from build123d import *

# Parameters (mm, degrees)
F0_R          = 14.5
F2_R          = 12.5
F5_R          = 10.8
F4_R          = 12.8
F8_R          = 14.5
F8_R_2        = 12.25
F9_DEPTH      = 0.5
F10_DEPTH     = 0.5
F11_R         = 0.2
F13_R         = 14
F13_R_2       = 12.2
F14_DEPTH     = 0.5
F15_DEPTH     = 0.5
F16_W         = 3
F16_H         = 15
F16_H_2       = 3
F16_W_2       = 15
F17_DEPTH     = 10
F18_T2_ANGLE  = 82.921707092
F18_T4_ANGLE  = 82.921707092
F18_T6_ANGLE  = 82.921707092
F18_T8_ANGLE  = 82.921707092
F18_T10_ANGLE = 82.921707092
F18_T12_ANGLE = 82.921707092
F18_T14_ANGLE = 82.921707092
F18_T16_ANGLE = 82.921707092


# Not quite as in the source:
# - a fillet or chamfer that OpenCascade refuses, or shapes differently, is made with other operations: its cross-section is extruded or revolved along the edge and cut away or added
# - a feature of the source that left no trace in its solid (it failed there, or was rolled back) is left out


with BuildPart() as f3:
    # F0 (on Top) → F3 section 0
    with BuildSketch(Plane.XY):
        Circle(F0_R)
    # F2 (on offset) → F3 section 1
    with BuildSketch(Plane.XY.offset(90)):
        Circle(F2_R)
    loft()

    # F5 (on face) → F6 section 0
    with BuildSketch(Plane.XY.offset(90)):
        Circle(F5_R)
    # F4 (on Top) → F6 section 1
    with BuildSketch(Plane.XY):
        Circle(F4_R)
    loft(mode=Mode.SUBTRACT)

    # F8 (on offset) → F9 (cut)
    with BuildSketch(Plane.XY.offset(81)):
        Circle(F8_R)
        Circle(F8_R_2, mode=Mode.SUBTRACT)
    extrude(amount=F9_DEPTH, mode=Mode.SUBTRACT)

    # F8 (on offset) → F10 (cut)
    with BuildSketch(Plane.XY.offset(81)):
        Circle(F8_R)
        Circle(F8_R_2, mode=Mode.SUBTRACT)
    extrude(amount=-F10_DEPTH, mode=Mode.SUBTRACT)

    # F11
    f11_edges = [f3.edges().sort_by_distance(p)[0] for p in [
        (-12.711111, 0, 80.5),
        (-12.688889, 0, 81.5),
    ]]
    fillet(f11_edges, radius=F11_R)

    # F13 (on offset) → F14 (join)
    with BuildSketch(Plane.XY.offset(3)):
        Circle(F13_R)
        Circle(F13_R_2, mode=Mode.SUBTRACT)
    extrude(amount=F14_DEPTH)

    # F13 (on offset) → F15 (join)
    with BuildSketch(Plane.XY.offset(3)):
        Circle(F13_R)
        Circle(F13_R_2, mode=Mode.SUBTRACT)
    extrude(amount=F15_DEPTH)

    # F16 (on face) → F17 (cut)
    with BuildSketch(Plane.XY):
        with Locations((0, 9)):
            Rectangle(F16_W, F16_H)
        Rectangle(F16_W, F16_H_2)
        with Locations((-9, 0)):
            Rectangle(F16_W_2, F16_H_2)
        with Locations((9, 0)):
            Rectangle(F16_W_2, F16_H_2)
        with Locations((0, -9)):
            Rectangle(F16_W, F16_H)
    extrude(amount=F17_DEPTH, mode=Mode.SUBTRACT)

    # F18: fillet of radius 0.3 on 8 edges, made by hand

    # F18_s1 → F18_t2 (revolve, cut)
    with BuildSketch(Plane(origin=(0, 0, 0), x_dir=(0, 0, 1), z_dir=(-0.0617304854, 0.998092855, 0))):
        with BuildLine():
            ThreePointArc((3.3, -12.2), (3.0878679656, -12.2878679656), (3, -12.5))
            Line((3, -12.5), (3, -12.2))
            Line((3, -12.2), (3.3, -12.2))
        make_face()
    revolve(axis=Axis((0, 0, 3), (0, 0, 1)), revolution_arc=F18_T2_ANGLE, mode=Mode.SUBTRACT)

    # F18_s3 → F18_t4 (revolve, cut)
    with BuildSketch(Plane(origin=(0, 0, 0), x_dir=(0, 0, 1), z_dir=(-0.0617304854, 0.998092855, 0))):
        with BuildLine():
            ThreePointArc((3.5, -12.5), (3.4121320344, -12.2878679656), (3.2, -12.2))
            Line((3.2, -12.2), (3.5, -12.2))
            Line((3.5, -12.2), (3.5, -12.5))
        make_face()
    revolve(axis=Axis((0, 0, 3.5), (0, 0, 1)), revolution_arc=F18_T4_ANGLE, mode=Mode.SUBTRACT)

    # F18_s5 → F18_t6 (revolve, cut)
    with BuildSketch(Plane(origin=(0, 0, 0), x_dir=(0, 0, 1), z_dir=(-0.998092855, -0.0617304854, 0))):
        with BuildLine():
            ThreePointArc((3.3, -12.2), (3.0878679656, -12.2878679656), (3, -12.5))
            Line((3, -12.5), (3, -12.2))
            Line((3, -12.2), (3.3, -12.2))
        make_face()
    revolve(axis=Axis((0, 0, 3), (0, 0, 1)), revolution_arc=F18_T6_ANGLE, mode=Mode.SUBTRACT)

    # F18_s7 → F18_t8 (revolve, cut)
    with BuildSketch(Plane(origin=(0, 0, 0), x_dir=(0, 0, 1), z_dir=(-0.998092855, -0.0617304854, 0))):
        with BuildLine():
            ThreePointArc((3.5, -12.5), (3.4121320344, -12.2878679656), (3.2, -12.2))
            Line((3.2, -12.2), (3.5, -12.2))
            Line((3.5, -12.2), (3.5, -12.5))
        make_face()
    revolve(axis=Axis((0, 0, 3.5), (0, 0, 1)), revolution_arc=F18_T8_ANGLE, mode=Mode.SUBTRACT)

    # F18_s9 → F18_t10 (revolve, cut)
    with BuildSketch(Plane(origin=(0, 0, 0), x_dir=(0, 0, 1), z_dir=(0.0617304854, -0.998092855, 0))):
        with BuildLine():
            ThreePointArc((3.3, -12.2), (3.0878679656, -12.2878679656), (3, -12.5))
            Line((3, -12.5), (3, -12.2))
            Line((3, -12.2), (3.3, -12.2))
        make_face()
    revolve(axis=Axis((0, 0, 3), (0, 0, 1)), revolution_arc=F18_T10_ANGLE, mode=Mode.SUBTRACT)

    # F18_s11 → F18_t12 (revolve, cut)
    with BuildSketch(Plane(origin=(0, 0, 0), x_dir=(0, 0, 1), z_dir=(0.0617304854, -0.998092855, 0))):
        with BuildLine():
            ThreePointArc((3.5, -12.5), (3.4121320344, -12.2878679656), (3.2, -12.2))
            Line((3.2, -12.2), (3.5, -12.2))
            Line((3.5, -12.2), (3.5, -12.5))
        make_face()
    revolve(axis=Axis((0, 0, 3.5), (0, 0, 1)), revolution_arc=F18_T12_ANGLE, mode=Mode.SUBTRACT)

    # F18_s13 → F18_t14 (revolve, cut)
    with BuildSketch(Plane(origin=(0, 0, 0), x_dir=(0, 0, 1), z_dir=(0.998092855, 0.0617304854, 0))):
        with BuildLine():
            ThreePointArc((3.3, -12.2), (3.0878679656, -12.2878679656), (3, -12.5))
            Line((3, -12.5), (3, -12.2))
            Line((3, -12.2), (3.3, -12.2))
        make_face()
    revolve(axis=Axis((0, 0, 3), (0, 0, 1)), revolution_arc=F18_T14_ANGLE, mode=Mode.SUBTRACT)

    # F18_s15 → F18_t16 (revolve, cut)
    with BuildSketch(Plane(origin=(0, 0, 0), x_dir=(0, 0, 1), z_dir=(0.998092855, 0.0617304854, 0))):
        with BuildLine():
            ThreePointArc((3.5, -12.5), (3.4121320344, -12.2878679656), (3.2, -12.2))
            Line((3.2, -12.2), (3.5, -12.2))
            Line((3.5, -12.2), (3.5, -12.5))
        make_face()
    revolve(axis=Axis((0, 0, 3.5), (0, 0, 1)), revolution_arc=F18_T16_ANGLE, mode=Mode.SUBTRACT)


solid = f3.part
The listing builds one solid part. Answer for the finished solid, in the listing's coordinates (mm). A direction names the side the tool comes from. Give positions to 0.01 mm unless a question says otherwise; leave off trailing zeros. Loops run counter-clockwise (first coordinate to the right, second up) from the corner with the lowest first, then second, coordinate; pieces in that order, holes last.
Item 1: A cutting plane is placed at A-A (x = 0). Give the vertices of the cut face in (y, z).
Derived:
outline: (-14.28, 10) - (-12.58, 10) - (-10.8, 90) - (-12.5, 90) - (-12.68, 81.7) arc R0.2 ccw to (-12.48, 81.5) - (-12.25, 81.5) - (-12.25, 80.5) - (-12.52, 80.5) arc R0.2 ccw to (-12.72, 80.3) - close; (10.8, 90) - (12.58, 10) - (14.28, 10) - (12.72, 80.3) arc R0.2 ccw to (12.52, 80.5) - (12.25, 80.5) - (12.25, 81.5) - (12.48, 81.5) arc R0.2 ccw to (12.68, 81.7) - (12.5, 90) - close
Item 2: A tool of negligible diameter and unlimited length cuts with its end or side. For faces 1 (the flat face through (14, 1.5, 5)), 2 (the conical face through (-9.112, -8.943, 1.479)), 3 (the conical face through (-9.28, 8.51, 85.91)), 4 (the flat face through (0, -13, 10)), from which of +Z, -Z, +X, -X, +Y, -Y can it reach the whole face along a straight path? Write none if from no direction.
Derived:
face 1: -Z, +X, -X
face 2: -Z
face 3: +Z
face 4: -Z, +Y, -Y
Item 3: Find the intervals of material crossed by line 1 along X through (y, z) = (-4.5, 44); line 2 along Y through (x, z) = (2.75, 81); line 3 along Y through (x, z) = (6, 51), in increasing order.
Derived:
line 1: x = -12.75 to -10.93, 10.93 to 12.75
line 2: y = -11.94 to -10.65, 10.65 to 11.94
line 3: y = -11.94 to -10.01, 10.01 to 11.94
Item 4: A cutting plane is placed at B-B (z = 45). Give the vertices of the cut face in (x, y), then the cut area to 3 significant figures.
Derived:
outline: circle Ø27 at (0, 0); hole circle Ø23.6 at (0, 0)
area: 135 mm2
Item 5: A cutting plane is placed at C-C (z = 55). Give the vertices of the cut face in (x, y).
Derived:
outline: circle Ø26.56 at (0, 0); hole circle Ø23.16 at (0, 0)
Item 6: Each of these flat-tipped pins is pushed along its axis until it touches: pin 1 Ø2 at (x, y) = (0, -13) entering from -Z; pin 2 Ø8 at (x, z) = (-6.5, 27.5) entering from +Y; pin 3 Ø6 at (y, z) = (8.5, 73) entering from -X; pin 4 Ø2 at (x, y) = (8.5, -2.5) entering from -Z. Where does it stop, or does it pass through?
Derived:
pin 1: stops at z = 10
pin 2: stops at y = 13.67
pin 3: stops at x = -11.65
pin 4: passes through
